Autodesk Inventor part; units mm, degrees
ref_plane "YZ Plane" through (0, 0, 0) normal (1, 0, 0) x (0, 1, 0)
ref_plane "XZ Plane" through (0, 0, 0) normal (0, 1, 0) x (-1, 0, 0)
ref_plane "XY Plane" through (0, 0, 0) normal (0, 0, 1) x (1, 0, 0)
sketch "Boceto1" plane through (0, 0, 0) normal (0, 0, 1) x (1, 0, 0)
  line L0 (0, 0) -> (0, 15.2)
  line L1 (0, 15.2) -> (9.6, 15.2)
  line L2 (0, 0) -> (9.6, 0)
  line L3 (9.6, 0) -> (14.6, 0) construction
  line L4 (14.6, 0) -> (24.6, 0) construction
  line L5 (24.6, 0) -> (24.6, 3) construction
  line L6 (24.6, 3) -> (14.2, 3)
  line L7 (14.2, 3) -> (9.6, 0)
  line L8 (24.6, 3) -> (24.6, 12.2)
  line L9 (24.6, 12.2) -> (14.2, 12.2)
  line L10 (14.2, 12.2) -> (9.6, 15.2)
  line L11 (49.2, 0) -> (49.2, 15.2)
  line L12 (49.2, 15.2) -> (39.6, 15.2)
  line L13 (49.2, 0) -> (39.6, 0)
  line L14 (39.6, 0) -> (34.6, 0) construction
  line L15 (34.6, 0) -> (24.6, 0) construction
  line L16 (24.6, 3) -> (35, 3)
  line L17 (35, 3) -> (39.6, 0)
  line L18 (24.6, 12.2) -> (35, 12.2)
  line L19 (35, 12.2) -> (39.6, 15.2)
  dimension "d0" = 15.2
  dimension "d1" = 9.6
  dimension "d2" = 9.6
  dimension "d3" = 5
  dimension "d4" = 10
  dimension "d5" = 3
  dimension "d6" = 10.4
  dimension "d7" = 9.2
  dimension "d8" = 10.4
extrude "Extrusión1" add sketch "Boceto1" along normal blind 15
equation "\"d4\" = Largo_seccion"
equation "\"d5\" = Espesor_centro"
equation "\"Largo_seccion\" = 10"
equation "\"Espesor_centro\" = 3"
properties part number "Spline_parametrizado"
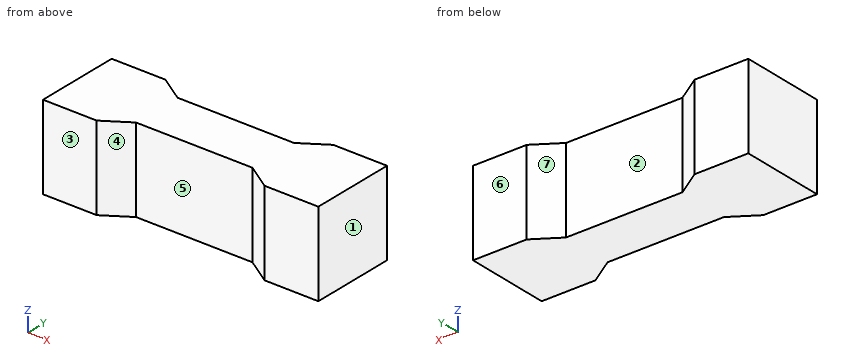
Can you work these out from the model? Positions are in its coordinate system, mm. Face numbers are marked on the shaded views. A direction names the side the tool comes from. Give positions to 0.01 mm unless a question says otherwise; leave off trailing zeros. Loops run counter-clockwise (first coordinate to the right, second up) from the corner with the lowest first, then second, coordinate; pieces in that order, holes last. Notation, with made-up numbers: (-3, 37.25) - (19, 37.25) arc R31 cw to (19, 70.25) - close; hole circle Ø3 at (-18, 59). An arc over 180 degrees is marked (long way). One line per item, written item: value.
(1) If we section it at C-C, the plane y = 12.75: List the corners of the cut face in (x, z) for me, plus the area to 3 significant figures.
Verdict:
outline: (0, 0) - (13.36, 0) - (13.36, 15) - (0, 15) - close; (35.84, 0) - (49.2, 0) - (49.2, 15) - (35.84, 15) - close
area: 401 mm^2
(2) If we section it at A-A, the plane y = 14.75: List the corners of the cut face in (x, z) for me.
Verdict:
outline: (0, 0) - (10.29, 0) - (10.29, 15) - (0, 15) - close; (38.91, 0) - (49.2, 0) - (49.2, 15) - (38.91, 15) - close
(3) I'm going to push flat-ended pins straight in: pin 1 (4.5 mm diameter, centred on x = 20, z = 4, fed in from -Y); pin 2 (2 mm diameter, centred on y = 10.5, z = 8, fed in from -X). Where does each tip first touch, or does it pass through?
Verdict:
pin 1: y = 3
pin 2: x = 0
(4) I need wall thicknesses on line 1 along Y through (x, z) = (31, 13.5); line 2 along X through (y, z) = (13.25, 9.5); line 3 along X through (y, z) = (14.25, 2). Which ranges of each line are inside material? Lowest first, please.
Verdict:
line 1: 3 to 12.2
line 2: 0 to 12.59, 36.61 to 49.2
line 3: 0 to 11.06, 38.14 to 49.2
(5) If we section it at D-D, the plane x = 26: List the corners of the cut face in (y, z) for me, plus the area to 3 significant figures.
Verdict:
outline: (3, 0) - (12.2, 0) - (12.2, 15) - (3, 15) - close
area: 138 mm^2
(6) If we section it at B-B, the plane z = 7.25: List the corners of the cut face in (x, y) for me.
Verdict:
outline: (0, 0) - (9.6, 0) - (14.2, 3) - (35, 3) - (39.6, 0) - (49.2, 0) - (49.2, 15.2) - (39.6, 15.2) - (35, 12.2) - (14.2, 12.2) - (9.6, 15.2) - (0, 15.2) - close
(7) If we mould it in two halves opening along X, with no side actions, what happens to the marked faces 1, 2, 3 and 4? For each: released by +X, released by -X, zero draft, split by the parting line, or undercut.
Verdict:
face 1: released by +X
face 2: undercut
face 3: zero draft
face 4: undercut
(8) On a 3-axis mill with a long thin cutter (end or side, diameter ignored), from which of +Z, -Z, +X, -X, +Y, -Y can I reach the whole of each face in a straight line? I mean the marked faces 5, 6 and 7. Say none if no direction works.
Verdict:
face 5: +Z, -Z, -Y
face 6: +Z, -Z, +X, -X, +Y
face 7: +Z, -Z, +Y
